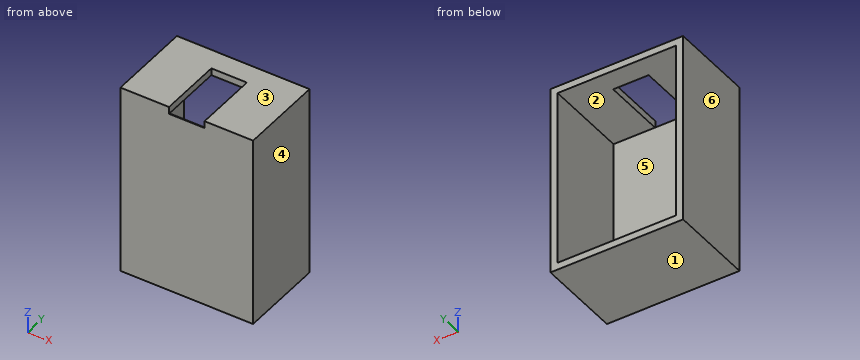
```python
from build123d import *

# Parameters (mm, degrees)
SKETCH1_W           = 474.133333334
SKETCH1_H           = 685.8
SKETCH1_W_2         = 423.333333334
SKETCH1_H_2         = 635
EXTRUDE_THIN1_DEPTH = 304.8
SKETCH1_2_W         = 423.333333334
SKETCH1_2_H         = 635
BOSS_EXTRUDE1_DEPTH = 2.54
SKETCH2_W           = 127
SKETCH2_H           = 228.6
CUT_EXTRUDE1_DEPTH  = 25.4


with BuildPart() as part:
    # Sketch1 → Extrude-Thin1 (new body)
    with BuildSketch(Plane(origin=(0, 0, 0), x_dir=(1, 0, 0), z_dir=(0, 1, 0))):
        Rectangle(SKETCH1_W, SKETCH1_H)
        Rectangle(SKETCH1_W_2, SKETCH1_H_2, mode=Mode.SUBTRACT)
    extrude(amount=EXTRUDE_THIN1_DEPTH)

    # Sketch1<2> → Boss-Extrude1 (add)
    with BuildSketch(Plane(origin=(0, 0, 0), x_dir=(1, 0, 0), z_dir=(0, 1, 0))):
        Rectangle(SKETCH1_2_W, SKETCH1_2_H)
    extrude(amount=BOSS_EXTRUDE1_DEPTH)

    # Sketch2 → Cut-Extrude1 (cut)
    with BuildSketch(Plane.XY.offset(342.9)):
        with Locations((0, 114.3)):
            Rectangle(SKETCH2_W, SKETCH2_H)
    extrude(amount=-CUT_EXTRUDE1_DEPTH, mode=Mode.SUBTRACT)


solid = part.part
```
Build history of the part. All positions in model axes, mm. Face numbers are marked on the shaded views. A direction names the side the tool comes from. Round coordinates to 2 decimals unless told otherwise and drop trailing zeros. Loops run counter-clockwise (first coordinate to the right, second up) from the corner with the lowest first, then second, coordinate; pieces in that order, holes last.
Item 1: Which spindle directions (+Z, -Z, +X, -X, +Y, -Y) get a long thin tool onto all of the face, cutting with end or side? Do the marked faces 5 and 6. Say none if no direction does.
Item 2: Saw through at B-B (x = 46). List the corners of the cut face in (y, z), then the cut area to 3 significant figures.
Item 3: Drill centre lines: line 1 along X through (y, z) = (194, 235); line 2 along Z through (x, y) = (138.5, 68); line 3 along Y through (x, z) = (-132, 2.5). Where is each one in solid material? Low to high.
Item 4: Saw through at C-C (z = -60). List the corners of the cut face in (x, y).
Item 5: Two-plate mould, pull along Z, no slides. Class the marked faces 1, 2, 3 and 4: released by +Z, released by -Z, zero draft, split by the parting line, or undercut.
Item 6: Pin check, flat tips, straight feed: P1, Ø1, axis at x = 186.5, z = -159, coming from the +Y side; P2, Ø12.5, axis at x = -21, z = 329.5, coming from the -Y side; P3, Ø2, axis at x = 13.5, y = 2, coming from the +Z side. Stop position of each tip, or through.
Item 7: Saw through at A-A (y = 278.5). List the corners of the cut face in (x, z).
Item 8: Saw through at D-D (y = 46). List the corners of the cut face in (x, z).
Worked answers:
1. face 5: +Y
1. face 6: +Z, -Z, -X, +Y, -Y
2. outline: (0, -342.9) - (304.8, -342.9) - (304.8, -317.5) - (2.54, -317.5) - (2.54, 317.5) - (0, 317.5) - close; (228.6, 317.5) - (304.8, 317.5) - (304.8, 342.9) - (228.6, 342.9) - close
2. area: 11,300 mm2
3. line 1: x = -237.07 to -211.67, 211.67 to 237.07
3. line 2: z = -342.9 to -317.5, 317.5 to 342.9
3. line 3: y = 0 to 2.54
4. outline: (-237.07, 0) - (237.07, 0) - (237.07, 304.8) - (211.67, 304.8) - (211.67, 2.54) - (-211.67, 2.54) - (-211.67, 304.8) - (-237.07, 304.8) - close
5. face 1: released by -Z
5. face 2: undercut
5. face 3: released by +Z
5. face 4: zero draft
6. P1: stops at y = 2.54
6. P2: stops at y = 228.6
6. P3: stops at z = 317.5
7. outline: (-237.07, -342.9) - (237.07, -342.9) - (237.07, 342.9) - (-237.07, 342.9) - close; hole (-211.67, -317.5) - (211.67, -317.5) - (211.67, 317.5) - (-211.67, 317.5) - close
8. outline: (-237.07, -342.9) - (237.07, -342.9) - (237.07, 342.9) - (63.5, 342.9) - (63.5, 317.5) - (211.67, 317.5) - (211.67, -317.5) - (-211.67, -317.5) - (-211.67, 317.5) - (-63.5, 317.5) - (-63.5, 342.9) - (-237.07, 342.9) - close
